Check sheet for the drawn part. Datum: minimum x, y, z corner. Units: mm. Round coordinates to 2 decimals unless told otherwise and drop trailing zeros. Write each loop counter-clockwise with the first axis right and the second up, starting at its lowest first coordinate (ties: lowest second). Pieces come first, ordered by that corner, then holes. Notation, with made-up numbers: M 81.25,89 L 102.25,89 A21 ccw 102.25,102 Z; hole C 63.5,2 d6. An arc over 180 degrees is marked long. Put each result on its own line as item: value.
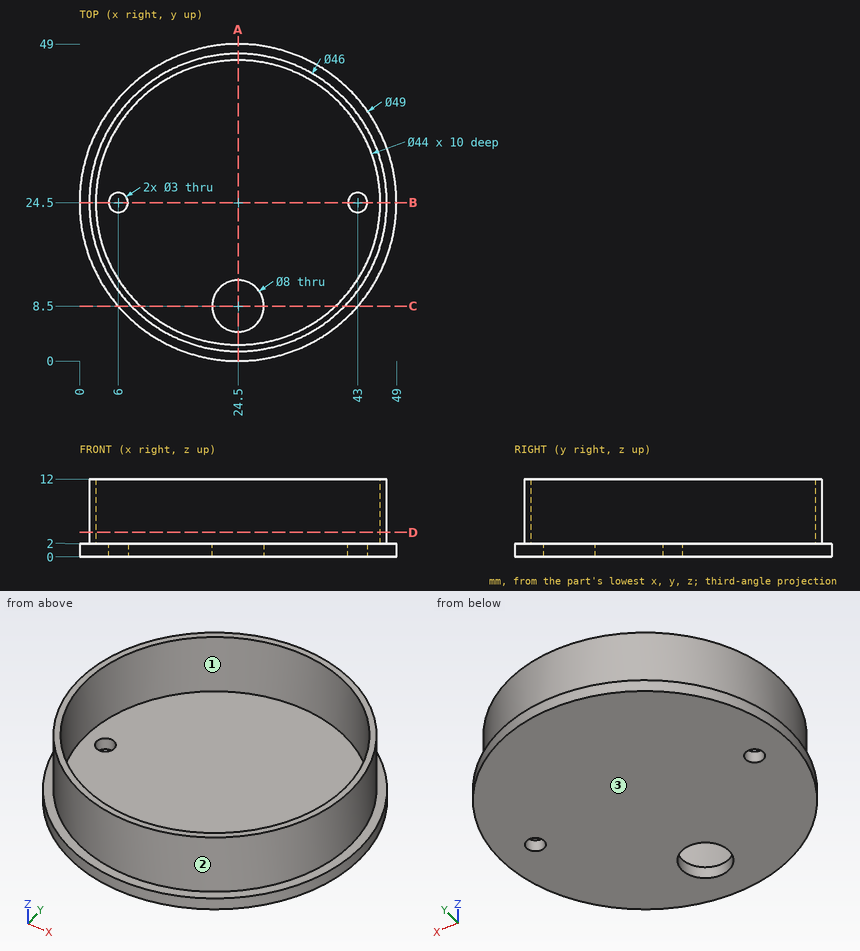
1. Cross-section at C-C (y = 8.5). Enter the section's corners in (x, z), then the cut area to 3 significant figures.
Computed values:
outline: M 5.95,0 L 20.5,0 L 20.5,2 L 9.4,2 L 9.4,12 L 7.98,12 L 7.98,2 L 5.95,2 Z; M 28.5,0 L 43.05,0 L 43.05,2 L 41.02,2 L 41.02,12 L 39.6,12 L 39.6,2 L 28.5,2 Z
area: 86.7 mm2
2. Release check for a two-part mould opening along Y. For the marked faces 1, 2 and 3 record: +Y half, -Y half, draft (parallel to the pull), parting line (faces both ways), or undercut.
Computed values:
face 1: undercut
face 2: parting line
face 3: draft
3. Scan lines: probe 1 along Y at (x, z) = (24.5, 1.55); probe 2 along Z at (x, y) = (22, 28); probe 3 along X at (y, z) = (33.5, 2.25). Record each from-to range of solid material in increasing order.
Computed values:
probe 1: y = 0 to 4.5, 12.5 to 49
probe 2: z = 0 to 2
probe 3: x = 3.33 to 4.43, 44.57 to 45.67
4. Cross-section at B-B (y = 24.5). Enter the section's corners in (x, z).
Computed values:
outline: M 0,0 L 4.5,0 L 4.5,2 L 2.5,2 L 2.5,12 L 1.5,12 L 1.5,2 L 0,2 Z; M 7.5,0 L 41.5,0 L 41.5,2 L 7.5,2 Z; M 44.5,0 L 49,0 L 49,2 L 47.5,2 L 47.5,12 L 46.5,12 L 46.5,2 L 44.5,2 Z
5. Cross-section at D-D (z = 3.75). Enter the section's corners in (x, y).
Computed values:
outline: C 24.5,24.5 d46; hole C 24.5,24.5 d44
6. Depth check by flat-ended pin: pin 1 Ø9 at (x, y) = (24.5, 8.5) entering from +Z; pin 2 Ø4 at (x, z) = (9.5, 7) entering from -Y; pin 3 Ø3 at (y, z) = (32.5, 5.5) entering from +X. Enter the tip coordinate at first touch or a pass-through.
Computed values:
pin 1: stops at z = 2
pin 2: stops at y = 5.53
pin 3: stops at x = 46.56
7. Cross-section at A-A (x = 24.5). Enter the section's corners in (y, z).
Computed values:
outline: M 0,0 L 4.5,0 L 4.5,2 L 2.5,2 L 2.5,12 L 1.5,12 L 1.5,2 L 0,2 Z; M 12.5,0 L 49,0 L 49,2 L 47.5,2 L 47.5,12 L 46.5,12 L 46.5,2 L 12.5,2 Z
